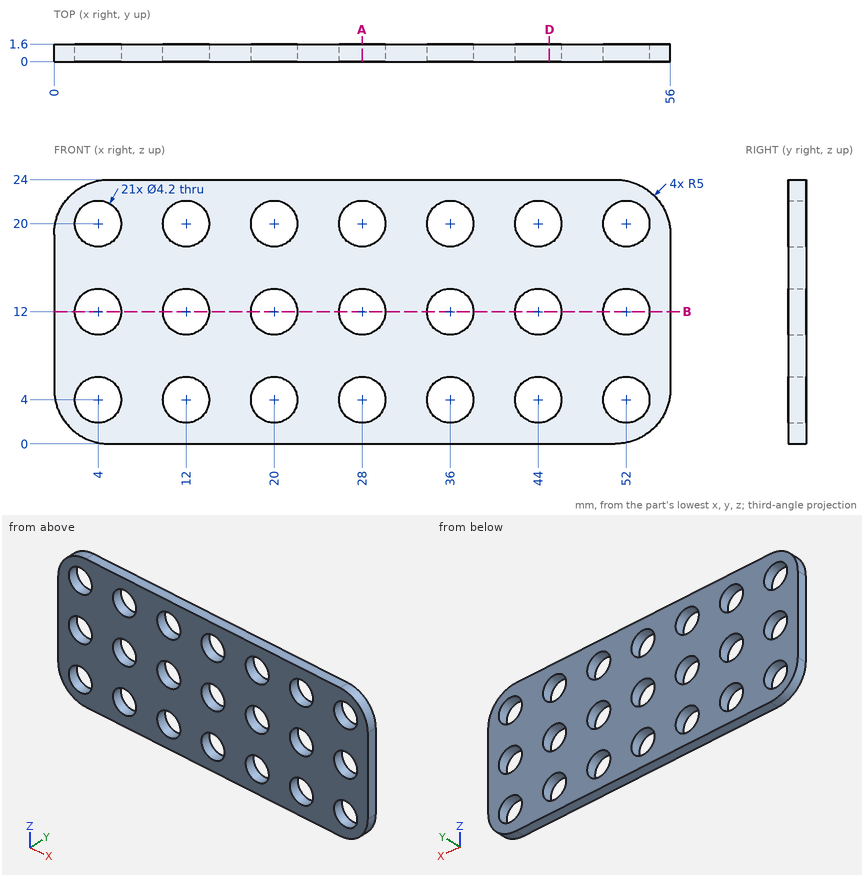
Input: dimensioned drawing with shaded views. Units: mm. Origin: part minimum x, y, z. Round coordinates to 2 decimals unless told otherwise and drop trailing zeros. Order: outer loops, then holes, each group sorted by start corner. A loop starts at its lowest first (then second) coordinate and runs counter-clockwise, first axis right, second up. Notation, with made-up numbers: M 83.5,53 L 99.5,53 A23 cw 99.5,70 Z; hole C 78.5,81.5 d1. An arc over 180 degrees is marked long. Use one line per item in the form item = value. Start each with the question number.
Q1. Pin query (flat end, axial travel): pin 1 Ø6.5 at (x, z) = (52, 4) entering from -Y. Return the tip coordinate at first contact, or that it passes through.
Q2. Material intervals for line 1 (Z direction, x = 20, y = 0.7); line 2 (Z direction, x = 5.5, y = 1.45), sorted ascending. Write a range as [from, to].
Q3. Cut plane A-A (x = 28). Return loops of the section in (y, z).
Q4. Cut plane B-B (z = 12). Count the separate pieces of the cut face and the enclosed holes in it, and give its area (3 significant figures).
Q5. Cut plane D-D (x = 45). Return loops of the section in (y, z), and give its area (3 significant figures).
Geometry results:
q1.pin_1 = 0
q2.line_1 = [0, 1.9], [6.1, 9.9], [14.1, 17.9], [22.1, 24]
q2.line_2 = [0, 2.53], [5.47, 10.53], [13.47, 18.53], [21.47, 24]
q3.outline = M 0,0 L 1.6,0 L 1.6,1.9 L 0,1.9 Z; M 0,6.1 L 1.6,6.1 L 1.6,9.9 L 0,9.9 Z; M 0,14.1 L 1.6,14.1 L 1.6,17.9 L 0,17.9 Z; M 0,22.1 L 1.6,22.1 L 1.6,24 L 0,24 Z
q4.separate_pieces = 8
q4.enclosed_holes = 0
q4.area = 42.6 mm^2
q5.outline = M 0,0 L 1.6,0 L 1.6,2.15 L 0,2.15 Z; M 0,5.85 L 1.6,5.85 L 1.6,10.15 L 0,10.15 Z; M 0,13.85 L 1.6,13.85 L 1.6,18.15 L 0,18.15 Z; M 0,21.85 L 1.6,21.85 L 1.6,24 L 0,24 Z
q5.area = 20.7 mm^2
